Verification items for the finished model (mm, model axes). Face numbers are marked on the shaded views. Give positions to 0.01 mm unless a question says otherwise; leave off trailing zeros. Loops run counter-clockwise (first coordinate to the right, second up) from the corner with the lowest first, then second, coordinate; pieces in that order, holes last. Notation, with made-up numbers: (-6.5, 80) - (14.5, 80) arc R19 cw to (14.5, 86) - close; hole circle Ø5 at (-34.75, -22.5). An arc over 180 degrees is marked (long way). Use one line per item in the form item = value.
```python
from build123d import *

# Parameters (mm, degrees)
SKETCH_1_W      = 170
SKETCH_1_H      = 60
SKETCH_1_W_2    = 4.5
SKETCH_1_H_2    = 8
SKETCH_1_W_3    = 8
SKETCH_1_H_3    = 17
SKETCH_1_W_4    = 4
SKETCH_1_W_5    = 9
EXTRUDE_1_DEPTH = 3
SKETCH_2_R      = 2.5
EXTRUDE_2_DEPTH = 25
SKETCH_3_W      = 170
SKETCH_3_H      = 60
EXTRUDE_3_DEPTH = 5


with BuildPart() as part:
    # 草图1 → 凸台-拉伸1 (new body)
    with BuildSketch(Plane(origin=(0, 0, 0), x_dir=(1, 0, 0), z_dir=(0, 1, 0))):
        with Locations((29.55216782, -0.710346801)):
            Rectangle(SKETCH_1_W, SKETCH_1_H)
        with Locations((-32.22272899, 0.64083336)):
            Rectangle(SKETCH_1_W_2, SKETCH_1_H_2, mode=Mode.SUBTRACT)
        with Locations((-21.72272899, 0.64083336)):
            Rectangle(SKETCH_1_W_2, SKETCH_1_H_2, mode=Mode.SUBTRACT)
        with Locations((86.428168623, 0.64083336)):
            Rectangle(SKETCH_1_W_3, SKETCH_1_H_3, mode=Mode.SUBTRACT)
        with Locations((29.933311746, -6.150891768)):
            Rectangle(SKETCH_1_W_4, SKETCH_1_H_2, mode=Mode.SUBTRACT)
        with Locations((22.455458099, 6.849108232)):
            Rectangle(SKETCH_1_W_5, SKETCH_1_H_2, mode=Mode.SUBTRACT)
        with Locations((37.455458099, 6.849108232)):
            Rectangle(SKETCH_1_W_5, SKETCH_1_H_2, mode=Mode.SUBTRACT)
    extrude(amount=EXTRUDE_1_DEPTH)

    # 草图2 → 凸台-拉伸2 (add)
    with BuildSketch(Plane.XZ):
        with Locations(Location((-50.44783218, 25.710346801, 0), (0, 0, 90))):
            Circle(SKETCH_2_R)
        with Locations(Location((-50.44783218, -24.289653199, 0), (0, 0, 90))):
            Circle(SKETCH_2_R)
        with Locations(Location((109.721085394, -24.289653199, 0), (0, 0, 90))):
            Circle(SKETCH_2_R)
        with Locations(Location((109.721085394, 25.710346801, 0), (0, 0, 90))):
            Circle(SKETCH_2_R)
        with Locations(Location((29.636626607, 25.710346801, 0), (0, 0, 90))):
            Circle(SKETCH_2_R)
        with Locations(Location((29.636626607, -24.289653199, 0), (0, 0, 90))):
            Circle(SKETCH_2_R)
    extrude(amount=EXTRUDE_2_DEPTH)

    # 草图3 → 凸台-拉伸3 (add)
    with BuildSketch(Plane.XZ.offset(25)):
        with Locations((29.55216782, 0.710346801)):
            Rectangle(SKETCH_3_W, SKETCH_3_H)
    extrude(amount=EXTRUDE_3_DEPTH)


solid = part.part
```
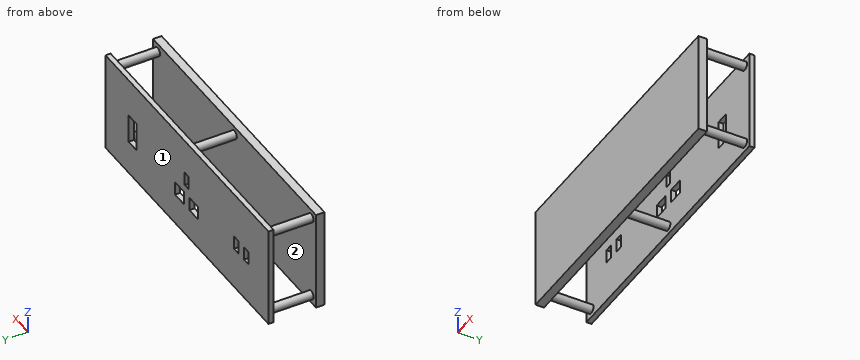
1. Draft check along X on the marked faces 1 and 2. Enter one of: released by +X, released by -X, zero draft, split by the parting line, or undercut.
Result set:
face_1 = zero draft
face_2 = undercut
2. Scan lines: probe 1 along Y at (x, z) = (70.5, -11); probe 2 along Z at (x, y) = (23, 0.5); probe 3 along X at (y, z) = (-2.5, 25). Record each from-to range of solid material in increasing order.
Result set:
probe_1 = -30 to -25, 0 to 3
probe_2 = -29.29 to -10.85, -2.85 to 30.71
probe_3 = -52.84 to -48.05, 27.24 to 32.03, 107.32 to 112.12
3. Section check B-B, the plane x = 100. Record the cut outline in (y, z).
Result set:
outline = (-30, -29.29) - (-25, -29.29) - (-25, 30.71) - (-30, 30.71) - close; (0, -29.29) - (3, -29.29) - (3, 30.71) - (0, 30.71) - close
4. Section check D-D, the plane y = -3. Record the cut outline in (x, z), then the cut area to 3 significant figures.
Result set:
outline = circle Ø5 at (-50.45, -24.29); circle Ø5 at (-50.45, 25.71); circle Ø5 at (29.64, -24.29); circle Ø5 at (29.64, 25.71); circle Ø5 at (109.72, -24.29); circle Ø5 at (109.72, 25.71)
area = 118 mm²
5. Section check C-C, the plane x = 24. Record the cut outline in (y, z).
Result set:
outline = (-30, -29.29) - (-25, -29.29) - (-25, 30.71) - (-30, 30.71) - close; (0, -29.29) - (3, -29.29) - (3, -10.85) - (0, -10.85) - close; (0, -2.85) - (3, -2.85) - (3, 30.71) - (0, 30.71) - close
6. Section check A-A, the plane z = 0. Record the cut outline in (x, y), then the cut area to 3 significant figures.
Result set:
outline = (-55.45, -30) - (114.55, -30) - (114.55, -25) - (-55.45, -25) - close; (-55.45, 0) - (-34.47, 0) - (-34.47, 3) - (-55.45, 3) - close; (-29.97, 0) - (-23.97, 0) - (-23.97, 3) - (-29.97, 3) - close; (-19.47, 0) - (82.43, 0) - (82.43, 3) - (-19.47, 3) - close; (90.43, 0) - (114.55, 0) - (114.55, 3) - (90.43, 3) - close
area = 1,310 mm²
7. Depth check by flat-ended pin: pin 1 Ø8 at (x, y) = (-24, -5) entering from +Z; pin 2 Ø3 at (x, y) = (34.5, -24.5) entering from +Z. Enter the tip coordinate at first touch or a pass-through.
Result set:
pin_1 = through
pin_2 = 30.71
